Autodesk Inventor part; units mm, degrees
ref_plane "YZ Plane" through (0, 0, 0) normal (1, 0, 0) x (0, 1, 0)
ref_plane "XZ Plane" through (0, 0, 0) normal (0, 1, 0) x (-1, 0, 0)
ref_plane "XY Plane" through (0, 0, 0) normal (0, 0, 1) x (1, 0, 0)
sketch "スケッチ1" plane through (0, 0, 0) normal (0, 0, 1) x (1, 0, 0)
  line L0 (0, 0) -> (23.2776, 0) construction
  line L1 (-7, -8.8) -> (7, -8.8)
  line L2 (7, -8.8) -> (7, -11.5)
  line L3 (7, -11.5) -> (-7, -11.5) construction
  line L4 (-7, -11.5) -> (-7, -8.8)
  line L5 (0, 0) -> (0, -16.4759) construction
  arc A0 (-7, -11.5) -> (7, -11.5) centre (0, 23.15) ccw
  line L6 (0, -12.2) -> (12.7013, -12.2) construction
  line L7 (0, 0) -> (-18.8146, 0) construction
  dimension "d0" = 14
  dimension "d1" = 8.8
  dimension "d2" = 12.2
  dimension "d4" = 11.5
revolve "回転1" add sketch "スケッチ1" angle 240 mid plane about axis through (0, 0, 0) along (-1, 0, 0)
fillet "フィレット1" radius 2 2 edges at (7, -11.5, 0) (-7, -11.5, 0)
properties part number "11_027_SHOE_GRIP_RUBBER_R1" material "ゴム、シリコーン"
Verification items for the finished model (mm, model axes). Coordinates: 2 decimals unless noted, no trailing zeros. Use CSV: the item, a comma, the result in double quotes.
Q1. Mould release check, pull along Z, two halves, no side actions. Record for faces 1 (the flat face through (-0.098, 5.238, -9.073)), 2 (the flat face through (-7, -9, 0)), 3 (the flat face through (-0.098, 5.238, 9.073)): pulls with the +Z half, pulls with the -Z half, needs draft (parallel to the pull), parting line crosses it, or undercut.
Computed values:
face 1,"undercut"
face 2,"needs draft"
face 3,"undercut"
Q2. Go/stop test with flat-tipped pins: P1, Ø2, axis at x = 2, y = -0.5, coming from the -Z side; P2, Ø3, axis at y = -8, z = 8.5, coming from the -X side; P3, Ø3, axis at x = 5.5, y = -5, coming from the +Z side. Record where each tip stops, or that it passes through.
Computed values:
P1,"z = -12.18"
P2,"x = -6.97"
P3,"z = 11.29"
Q3. Thickness scan on line 1 along Z through (x, y) = (1, 0); line 2 along Y through (x, z) = (0.5, 0); line 3 along Z through (x, y) = (-1.5, 1). Record the ranges inside material, lowest first. Write a range as [from, to].
Computed values:
line 1,"[-12.19, -8.8], [8.8, 12.19]"
line 2,"[-12.2, -8.8]"
line 3,"[-12.13, -8.74], [8.74, 12.13]"
